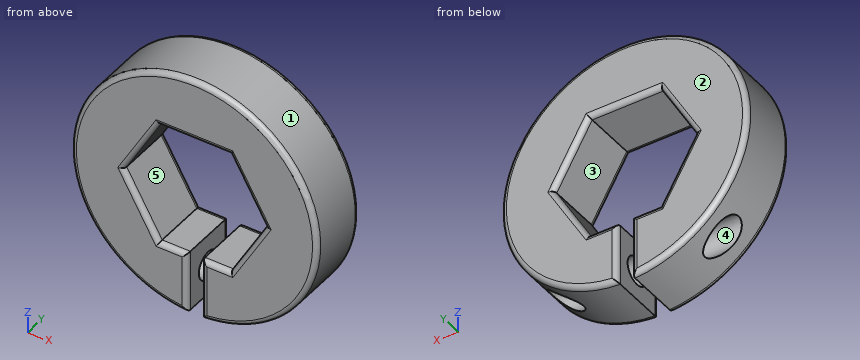
```python
from build123d import *

# Parameters (mm, degrees)
SKETCH1_R               = 12.7
BOSS_EXTRUDE1_DEPTH     = 6.35
SKETCH2_W               = 16.521892969
SKETCH2_H               = 16.064378343
CUT_EXTRUDE1_DEPTH      = 0.762
CUT_EXTRUDE1_DEPTH_BACK = 0.762
SKETCH3_R               = 1.450011988
CUT_EXTRUDE2_DEPTH      = 14.462
CUT_EXTRUDE2_DEPTH_BACK = 12.938
FILLET1_R               = 0.508


with BuildPart() as part:
    # Sketch1 → Boss-Extrude1 (new body)
    with BuildSketch(Plane(origin=(0, 0, 0), x_dir=(1, 0, 0), z_dir=(0, 1, 0))):
        Circle(SKETCH1_R)
        Polygon((7.332348419, 0), (3.666174209, 6.35), (-3.666174209, 6.35), (-7.332348419, 0), (-3.666174209, -6.35), (3.666174209, -6.35), align=None, mode=Mode.SUBTRACT)
    extrude(amount=BOSS_EXTRUDE1_DEPTH)

    # Sketch2 → Cut-Extrude1 (cut, two sides)
    with BuildSketch(Plane(origin=(0, 0, 0), x_dir=(0, 0, -1), z_dir=(1, 0, 0))) as cut_extrude1_sk:
        with Locations((10.843461422, 3.411156181)):
            Rectangle(SKETCH2_W, SKETCH2_H)
    extrude(amount=CUT_EXTRUDE1_DEPTH, mode=Mode.SUBTRACT)
    extrude(cut_extrude1_sk.sketch, amount=-CUT_EXTRUDE1_DEPTH_BACK, mode=Mode.SUBTRACT)

    # Sketch3 → Cut-Extrude2 (cut, two sides)
    with BuildSketch(Plane.ZY.offset(-0.762)) as cut_extrude2_sk:
        with Locations((-9.609846494, 3.271635)):
            Circle(SKETCH3_R)
    extrude(amount=CUT_EXTRUDE2_DEPTH, mode=Mode.SUBTRACT)
    extrude(cut_extrude2_sk.sketch, amount=-CUT_EXTRUDE2_DEPTH_BACK, mode=Mode.SUBTRACT)

    # Fillet1
    fillet1_edges = [part.edges().sort_by_distance(p)[0] for p in [
        (2.214087105, 0, -6.35),
        (-5.499261314, 0, -3.175),
        (-5.499261314, 0, 3.175),
        (0, 0, 6.35),
        (5.499261314, 6.35, 3.175),
        (5.499261314, 6.35, -3.175),
        (2.214087105, 6.35, -6.35),
        (-5.499261314, 6.35, -3.175),
        (-5.499261314, 6.35, 3.175),
        (0, 6.35, 6.35),
        (-2.214087105, 0, -6.35),
        (-2.214087105, 6.35, -6.35),
        (-8.706681343, 6.35, 9.245739559),
        (-8.706681343, 0, 9.245739559),
        (0.762, 0, -9.513559694),
        (-0.762, 6.35, -9.513559694),
        (0.762, 6.35, -9.513559694),
        (-0.762, 0, -9.513559694),
        (5.499261314, 0, 3.175),
        (5.499261314, 0, -3.175),
    ]]
    fillet(fillet1_edges, radius=FILLET1_R)


solid = part.part
```
Here's how the part is built. I have some questions about the finished solid (model axes, mm). Face numbers are marked on the shaded views. A direction names the side the tool comes from. Round coordinates to 2 decimals unless told otherwise and drop trailing zeros. Order: outer loops, then holes, each group sorted by start corner. A loop starts at its lowest first (then second) coordinate and runs counter-clockwise, first axis right, second up. Notation, with made-up numbers: (0, 63) -> (7, 63) arc R25 ccw to (7, 93) -> close; hole circle Ø6 at (34.5, 18). An arc over 180 degrees is marked (long way). Use a Markdown table: item, result. Add a question column.
(1) For pin 1 Ø12 at (x, z) = (0.5, 0.5) entering from -Y; pin 2 Ø2.5 at (y, z) = (3.27, -9.61) entering from -X; pin 3 Ø1.5 at (x, y) = (1.5, 2) entering from +Z; pin 4 Ø1.5 at (x, y) = (-2.5, 2) entering from +Z, each with a flat end and sliding along its axis, tell me the tip position at first contact or that it passes through.
(2) Suppose I cut it at B-B, the plane x = 0. Please give me the cut outline in (y, z).
(3) Suppose I cut it at C-C, the plane y = 2.5. Please give me the cut outline in (x, z), and give its area (3 significant figures).
(4) If we mould it in two halves opening along Z, with no side actions, what happens to the marked faces 1, 2 and 3? For each: released by +Z, released by -Z, zero draft, split by the parting line, or undercut.
(5) I need wall thicknesses on line 1 along Z through (x, y) = (-11, 4.5); line 2 along Z through (x, y) = (0.25, 5.25); line 3 along X through (y, z) = (0.5, -2.5). Which ranges of each line are inside material? Lowest first, please.
(6) For the marked faces 4 and 5, which set-ups out of +Z, -Z, +X, -X, +Y, -Y let a thin tool reach every point of the face, with its end or its side?
(7) Suppose I cut it at D-D, the plane x = 5. Count the separate pieces of the cut face and the enclosed holes in it, and give its area (3 significant figures).
(8) Suppose I cut it at A-A, the plane y = 5.25. Please give me the cut outline in (x, z), and give its area (3 significant figures).
Verdict:
| question | item | result |
|---|---|---|
| 1 | pin 1 | y = 0.03 |
| 1 | pin 2 | through |
| 1 | pin 3 | z = 12.68 |
| 1 | pin 4 | z = 12.58 |
| 2 | outline | (0, 6.86) arc R0.51 ccw to (0.51, 6.35) -> (5.84, 6.35) arc R0.51 ccw to (6.35, 6.86) -> (6.35, 12.19) arc R0.51 ccw to (5.84, 12.7) -> (0.51, 12.7) arc R0.51 ccw to (0, 12.19) -> close |
| 3 | outline | (-9.54, -8.38) -> (-0.76, -8.38) -> (-0.76, -6.35) -> (-3.67, -6.35) -> (-7.33, 0) -> (-3.67, 6.35) -> (3.67, 6.35) -> (7.33, 0) -> (3.67, -6.35) -> (0.76, -6.35) -> (0.76, -8.38) -> (9.54, -8.38) arc R12.7 ccw (long way) to start; (-6.62, -10.84) arc R12.7 ccw to (-0.76, -12.68) -> (-0.76, -10.84) -> close; (0.76, -12.68) arc R12.7 ccw to (6.62, -10.84) -> (0.76, -10.84) -> close |
| 3 | area | 321 mm2 |
| 4 | face 1 | split by the parting line |
| 4 | face 2 | zero draft |
| 4 | face 3 | undercut |
| 5 | line 1 | -6.35 to 6.35 |
| 5 | line 2 | 6.35 to 12.7 |
| 5 | line 3 | -12.45 to -5.89, 5.89 to 12.45 |
| 6 | face 4 | +X, -X |
| 6 | face 5 | +Y, -Y |
| 7 | separate pieces | 2 |
| 7 | enclosed holes | 1 |
| 7 | area | 89.7 mm2 |
| 8 | outline | (-7.33, 0) -> (-3.67, 6.35) -> (3.67, 6.35) -> (7.33, 0) -> (3.67, -6.35) -> (0.76, -6.35) -> (0.76, -12.68) arc R12.7 ccw (long way) to (-0.76, -12.68) -> (-0.76, -6.35) -> (-3.67, -6.35) -> close |
| 8 | area | 357 mm2 |
